Build history of the part. All positions in model axes, mm. A direction names the side the tool comes from. Give positions to 0.01 mm unless a question says otherwise; leave off trailing zeros. Order: outer loops, then holes, each group sorted by start corner. A loop starts at its lowest first (then second) coordinate and runs counter-clockwise, first axis right, second up. Notation, with made-up numbers: M 60,61.25 L 75,61.25 A29 cw 75,84.25 Z; hole C 59,30 d11. An arc over 180 degrees is marked long. Use CSV: the item, a comma, the result in double quotes. Start each with the question number.
Item 1: Which spindle directions (+Z, -Z, +X, -X, +Y, -Y) get a long thin tool onto all of the face, cutting with end or side? Do faces 4 (the cylindrical face through (58.995, 31.234, 40.742)), 5 (the cylindrical face through (-45.5, -28.2, -0.3)), 6 (the cylindrical face through (58.995, -31.234, -40.742)). Say none if no direction does.
Item 2: Band-saw the part on A-A on x = 0. Write the cut outline in (y, z).
Item 3: Wall check: line 1 along X through (y, z) = (28, -40); line 2 along Z through (x, y) = (53.5, -30.5); line 3 along X through (y, z) = (31.5, -39.5). Give the ranges that are in metal, low to high.
Item 4: Pin check, flat tips, straight feed: P1, Ø2, axis at y = -2.5, z = 62, coming from the -X side; P2, Ø5.5, axis at x = 53, z = 42, coming from the -Y side; P3, Ø3.5, axis at x = 53, z = 39.5, coming from the +Y side. Stop position of each tip, or through.
Item 5: Band-saw the part on C-C on y = 0. Write the cut outline in (x, z), plus the area to 3 significant figures.
Item 6: Band-saw the part on D-D on x = -43.5. Write the cut outline in (y, z).
Item 7: Two-plate mould, pull along Y, no slides. Class faces 1 (the flat face through (46, -37.15, -8)), 2 (the cylindrical face through (-53.258, -31.234, -45.995)), 3 (the cylindrical face through (-51.27, 17.73, 11.31)): pulls with the +Y half, pulls with the -Y half, needs draft (parallel to the pull), parting line crosses it, or undercut.
Item 8: Band-saw the part on B-B on z = 0. Write the cut outline in (x, y), plus the area to 3 significant figures.
from build123d import *

# Parameters (mm, degrees)
Y_KSEKLIK_EKSTR_ZYON1_DEPTH = 37.15
KES_EKSTR_ZYON1_DEPTH       = 74.3
IZIM3_R                     = 5.5
KES_EKSTR_ZYON2_DEPTH       = 12
DAIRESEL_KAPLAMA1_COUNT     = 5
DAIRESEL_KAPLAMA1_ANGLE     = 240
AYNALAMA1_COPY_1_SKETCH_R   = 5.5
AYNALAMA1_COPY_1_DEPTH      = 12
AYNALAMA1_COPY_2_SKETCH_R   = 5.5
AYNALAMA1_COPY_2_DEPTH      = 12
AYNALAMA1_COPY_3_SKETCH_R   = 5.5
AYNALAMA1_COPY_3_DEPTH      = 12
AYNALAMA1_COPY_4_SKETCH_R   = 5.5
AYNALAMA1_COPY_4_DEPTH      = 12
AYNALAMA2_COPY_1_SKETCH_R   = 5.5
AYNALAMA2_COPY_1_DEPTH      = 12
AYNALAMA2_COPY_2_SKETCH_R   = 5.5
AYNALAMA2_COPY_2_DEPTH      = 12
AYNALAMA2_COPY_3_SKETCH_R   = 5.5
AYNALAMA2_COPY_3_DEPTH      = 12
AYNALAMA2_COPY_4_SKETCH_R   = 5.5
AYNALAMA2_COPY_4_DEPTH      = 12
AYNALAMA2_COPY_5_SKETCH_R   = 5.5
AYNALAMA2_COPY_5_DEPTH      = 12
AYNALAMA2_COPY_6_SKETCH_R   = 5.5
AYNALAMA2_COPY_6_DEPTH      = 12
AYNALAMA2_COPY_7_SKETCH_R   = 5.5
AYNALAMA2_COPY_7_DEPTH      = 12
AYNALAMA2_COPY_8_SKETCH_R   = 5.5
AYNALAMA2_COPY_8_DEPTH      = 12
AYNALAMA2_COPY_9_SKETCH_R   = 5.5
AYNALAMA2_COPY_9_DEPTH      = 12
KES_EKSTR_ZYON3_REACH       = 166.052
KES_EKSTR_ZYON3_END_RADIUS  = 45.5
IZIM4_R                     = 21.03
KES_EKSTR_ZYON4_REACH       = 166.052
KES_EKSTR_ZYON4_END_RADIUS  = 45.5
IZIM5_R                     = 10.86


with BuildPart() as part:
    # Çizim1 → Yükseklik-Ekstrüzyon1 (new, symmetric)
    with BuildSketch(Plane(origin=(0, 0, 0), x_dir=(1, 0, 0), z_dir=(0, 1, 0))):
        with BuildLine():
            Line((61.5, 40.5), (61.5, -40.5))
            ThreePointArc((61.5, -40.5), (0, -102), (-61.5, -40.5))
            Line((-61.5, -40.5), (-61.5, 40.5))
            ThreePointArc((-61.5, 40.5), (0, 102), (61.5, 40.5))
        make_face()
    extrude(amount=Y_KSEKLIK_EKSTR_ZYON1_DEPTH, both=True)

    # Çizim2 → Kes-Ekstrüzyon1 (cut)
    with BuildSketch(Plane(origin=(0, 37.15, 0), x_dir=(1, 0, 0), z_dir=(0, 1, 0))):
        with BuildLine():
            ThreePointArc((40.745398513, 20.25), (0, 86), (-40.745398513, 20.25))
            ThreePointArc((-40.745398513, 20.25), (-45.5, 0), (-40.745398513, -20.25))
            ThreePointArc((-40.745398513, -20.25), (0, -86), (40.745398513, -20.25))
            ThreePointArc((40.745398513, -20.25), (45.5, 0), (40.745398513, 20.25))
        make_face()
    extrude(amount=-KES_EKSTR_ZYON1_DEPTH, mode=Mode.SUBTRACT)

    # Çizim3 → Kes-Ekstrüzyon2 (cut)
    with BuildSketch(Plane(origin=(0, 37.15, 0), x_dir=(1, 0, 0), z_dir=(0, 1, 0))):
        with Locations(Location((-53.5, 40.5, 0), (0, 0, 270))):
            Circle(IZIM3_R)
    kes_ekstr_zyon2 = extrude(amount=-KES_EKSTR_ZYON2_DEPTH, mode=Mode.SUBTRACT)

    # Dairesel Kaplama1: Kes-Ekstrüzyon2 ×5 about axis
    dairesel_kaplama1_axis = Axis((0, 0, -40.5), (0, -1, 0))
    for i in range(1, DAIRESEL_KAPLAMA1_COUNT):
        add(kes_ekstr_zyon2.rotate(dairesel_kaplama1_axis, i * DAIRESEL_KAPLAMA1_ANGLE / (DAIRESEL_KAPLAMA1_COUNT - 1)), mode=Mode.SUBTRACT)

    # Aynalama1: Kes-Ekstrüzyon2 across plane
    add(kes_ekstr_zyon2.mirror(Plane.XY), mode=Mode.SUBTRACT)

    # Aynalama1 copy 1 sketch → Aynalama1 copy 1 (cut)
    with BuildSketch(Plane(origin=(-35.074028853, 37.15, 20.25), x_dir=(0.4999999999999978, 0, -0.8660254037844399), z_dir=(0, 1, 0))):
        with Locations((-53.5, -40.5)):
            Circle(AYNALAMA1_COPY_1_SKETCH_R)
    extrude(amount=-AYNALAMA1_COPY_1_DEPTH, mode=Mode.SUBTRACT)

    # Aynalama1 copy 2 sketch → Aynalama1 copy 2 (cut)
    with BuildSketch(Plane(origin=(-35.074028853, 37.15, 60.75), x_dir=(-0.5000000000000044, 0, -0.866025403784436), z_dir=(0, 1, 0))):
        with Locations((-53.5, -40.5)):
            Circle(AYNALAMA1_COPY_2_SKETCH_R)
    extrude(amount=-AYNALAMA1_COPY_2_DEPTH, mode=Mode.SUBTRACT)

    # Aynalama1 copy 3 sketch → Aynalama1 copy 3 (cut)
    with BuildSketch(Plane(origin=(0, 37.15, 81), x_dir=(-1, 0, 0), z_dir=(0, 1, 0))):
        with Locations((-53.5, -40.5)):
            Circle(AYNALAMA1_COPY_3_SKETCH_R)
    extrude(amount=-AYNALAMA1_COPY_3_DEPTH, mode=Mode.SUBTRACT)

    # Aynalama1 copy 4 sketch → Aynalama1 copy 4 (cut)
    with BuildSketch(Plane(origin=(35.074028853, 37.15, 60.75), x_dir=(-0.4999999999999912, 0, 0.8660254037844437), z_dir=(0, 1, 0))):
        with Locations((-53.5, -40.5)):
            Circle(AYNALAMA1_COPY_4_SKETCH_R)
    extrude(amount=-AYNALAMA1_COPY_4_DEPTH, mode=Mode.SUBTRACT)

    # Aynalama2: Kes-Ekstrüzyon2 across plane
    add(kes_ekstr_zyon2.mirror(Plane.ZX), mode=Mode.SUBTRACT)

    # Aynalama2 copy 1 sketch → Aynalama2 copy 1 (cut)
    with BuildSketch(Plane(origin=(-35.074028853, -37.15, -20.25), x_dir=(0.4999999999999978, 0, 0.8660254037844399), z_dir=(0, -1, 0))):
        with Locations((-53.5, -40.5)):
            Circle(AYNALAMA2_COPY_1_SKETCH_R)
    extrude(amount=-AYNALAMA2_COPY_1_DEPTH, mode=Mode.SUBTRACT)

    # Aynalama2 copy 2 sketch → Aynalama2 copy 2 (cut)
    with BuildSketch(Plane(origin=(-35.074028853, -37.15, -60.75), x_dir=(-0.5000000000000044, 0, 0.866025403784436), z_dir=(0, -1, 0))):
        with Locations((-53.5, -40.5)):
            Circle(AYNALAMA2_COPY_2_SKETCH_R)
    extrude(amount=-AYNALAMA2_COPY_2_DEPTH, mode=Mode.SUBTRACT)

    # Aynalama2 copy 3 sketch → Aynalama2 copy 3 (cut)
    with BuildSketch(Plane(origin=(0, -37.15, -81), x_dir=(-1, 0, 0), z_dir=(0, -1, 0))):
        with Locations((-53.5, -40.5)):
            Circle(AYNALAMA2_COPY_3_SKETCH_R)
    extrude(amount=-AYNALAMA2_COPY_3_DEPTH, mode=Mode.SUBTRACT)

    # Aynalama2 copy 4 sketch → Aynalama2 copy 4 (cut)
    with BuildSketch(Plane(origin=(35.074028853, -37.15, -60.75), x_dir=(-0.4999999999999912, 0, -0.8660254037844437), z_dir=(0, -1, 0))):
        with Locations((-53.5, -40.5)):
            Circle(AYNALAMA2_COPY_4_SKETCH_R)
    extrude(amount=-AYNALAMA2_COPY_4_DEPTH, mode=Mode.SUBTRACT)

    # Aynalama2 copy 5 sketch → Aynalama2 copy 5 (cut)
    with BuildSketch(Plane.XZ.offset(37.15)):
        with Locations(Location((-53.5, 40.5, 0), (0, 0, 270))):
            Circle(AYNALAMA2_COPY_5_SKETCH_R)
    extrude(amount=-AYNALAMA2_COPY_5_DEPTH, mode=Mode.SUBTRACT)

    # Aynalama2 copy 6 sketch → Aynalama2 copy 6 (cut)
    with BuildSketch(Plane(origin=(-35.074028853, -37.15, 20.25), x_dir=(0.4999999999999978, 0, -0.8660254037844399), z_dir=(0, -1, 0))):
        with Locations(Location((-53.5, 40.5, 0), (0, 0, 270))):
            Circle(AYNALAMA2_COPY_6_SKETCH_R)
    extrude(amount=-AYNALAMA2_COPY_6_DEPTH, mode=Mode.SUBTRACT)

    # Aynalama2 copy 7 sketch → Aynalama2 copy 7 (cut)
    with BuildSketch(Plane(origin=(-35.074028853, -37.15, 60.75), x_dir=(-0.5000000000000044, 0, -0.866025403784436), z_dir=(0, -1, 0))):
        with Locations(Location((-53.5, 40.5, 0), (0, 0, 270))):
            Circle(AYNALAMA2_COPY_7_SKETCH_R)
    extrude(amount=-AYNALAMA2_COPY_7_DEPTH, mode=Mode.SUBTRACT)

    # Aynalama2 copy 8 sketch → Aynalama2 copy 8 (cut)
    with BuildSketch(Plane(origin=(0, -37.15, 81), x_dir=(-1, 0, 0), z_dir=(0, -1, 0))):
        with Locations(Location((-53.5, 40.5, 0), (0, 0, 270))):
            Circle(AYNALAMA2_COPY_8_SKETCH_R)
    extrude(amount=-AYNALAMA2_COPY_8_DEPTH, mode=Mode.SUBTRACT)

    # Aynalama2 copy 9 sketch → Aynalama2 copy 9 (cut)
    with BuildSketch(Plane(origin=(35.074028853, -37.15, 60.75), x_dir=(-0.4999999999999912, 0, 0.8660254037844437), z_dir=(0, -1, 0))):
        with Locations(Location((-53.5, 40.5, 0), (0, 0, 270))):
            Circle(AYNALAMA2_COPY_9_SKETCH_R)
    extrude(amount=-AYNALAMA2_COPY_9_DEPTH, mode=Mode.SUBTRACT)

    # Kes-Ekstrüzyon3: up to this cylinder (the profile starts outside it)
    kes_ekstr_zyon3_end = Plane(origin=(0, 0, 0), z_dir=(0, 1, 0)) * Cylinder(KES_EKSTR_ZYON3_END_RADIUS, 424.104, mode=Mode.PRIVATE)
    # Çizim4 → Kes-Ekstrüzyon3 (cut, up to the surface)
    with BuildSketch(Plane.ZY.offset(61.5), mode=Mode.PRIVATE) as kes_ekstr_zyon3_sk1:
        Circle(IZIM4_R)
    kes_ekstr_zyon3_tool1 = extrude(kes_ekstr_zyon3_sk1.sketch, amount=-KES_EKSTR_ZYON3_REACH, mode=Mode.PRIVATE) - kes_ekstr_zyon3_end
    add(kes_ekstr_zyon3_tool1.solids().sort_by_distance((-61.5, 0, 0))[0], mode=Mode.SUBTRACT)

    # Kes-Ekstrüzyon4: up to this cylinder (the profile starts outside it)
    kes_ekstr_zyon4_end = Plane(origin=(0, 0, 0), z_dir=(0, 1, 0)) * Cylinder(KES_EKSTR_ZYON4_END_RADIUS, 424.104, mode=Mode.PRIVATE)
    # Çizim5 → Kes-Ekstrüzyon4 (cut, up to the surface)
    with BuildSketch(Plane(origin=(61.5, 0, 0), x_dir=(0, 0, -1), z_dir=(1, 0, 0)), mode=Mode.PRIVATE) as kes_ekstr_zyon4_sk1:
        Circle(IZIM5_R)
    kes_ekstr_zyon4_tool1 = extrude(kes_ekstr_zyon4_sk1.sketch, amount=-KES_EKSTR_ZYON4_REACH, mode=Mode.PRIVATE) - kes_ekstr_zyon4_end
    add(kes_ekstr_zyon4_tool1.solids().sort_by_distance((61.5, 0, 0))[0], mode=Mode.SUBTRACT)


solid = part.part
Model answer:
1,face 4,"+Y"
1,face 5,"+Y, -Y"
1,face 6,"-Y"
2,outline,"M -37.15,-102 L 37.15,-102 L 37.15,-86 L -37.15,-86 Z; M -37.15,86 L 37.15,86 L 37.15,102 L -37.15,102 Z"
3,line 1,"x = -61.5 to -58.98, -48.02 to -45.5, 45.5 to 48.02, 58.98 to 61.5"
3,line 2,"z = -70.83 to -46, -35 to 35, 46 to 70.83"
3,line 3,"x = -61.5 to -58.91, -48.09 to -45.49, 45.49 to 48.09, 58.91 to 61.5"
4,P1,"stops at x = -57.98"
4,P2,"stops at y = -25.15"
4,P3,"stops at y = 25.15"
5,outline,"M -61.5,-40.5 A61.5 ccw 61.5,-40.5 L 61.5,-10.86 L 44.18,-10.86 A45.5 cw 40.75,-20.25 A45.5 cw long -41.12,-21.03 L -61.5,-21.03 Z; M -61.5,21.03 L -41.12,21.03 A45.5 cw long 40.75,20.25 A45.5 cw 44.18,10.86 L 61.5,10.86 L 61.5,40.5 A61.5 ccw -61.5,40.5 Z"
5,area,"7,120 mm^2"
6,outline,"M -37.15,-83.97 L 37.15,-83.97 L 37.15,-53.84 L -37.15,-53.84 Z; M -37.15,-27.16 L 37.15,-27.16 L 37.15,-13.34 L 16.26,-13.34 A21.03 cw -16.26,-13.34 L -37.15,-13.34 Z; M -37.15,13.34 L -16.26,13.34 A21.03 cw 16.26,13.34 L 37.15,13.34 L 37.15,27.16 L -37.15,27.16 Z; M -37.15,53.84 L 37.15,53.84 L 37.15,83.97 L -37.15,83.97 Z"
7,face 1,"pulls with the -Y half"
7,face 2,"needs draft"
7,face 3,"undercut"
8,outline,"M -61.5,-37.15 L -45.5,-37.15 L -45.5,-21.03 L -61.5,-21.03 Z; M -61.5,21.03 L -45.5,21.03 L -45.5,37.15 L -61.5,37.15 Z; M 45.5,-37.15 L 61.5,-37.15 L 61.5,-10.86 L 45.5,-10.86 Z; M 45.5,10.86 L 61.5,10.86 L 61.5,37.15 L 45.5,37.15 Z"
8,area,"1,360 mm^2"
